Part model, mm, in its own coordinate system. Face numbers are marked on the shaded views. A direction names the side the tool comes from. Coordinates: 2 decimals unless noted, no trailing zeros. Write each loop counter-clockwise with the first axis right and the second up, starting at its lowest first coordinate (ties: lowest second). Pieces come first, ordered by that corner, then holes. Notation, with made-up numbers: (32, 55.5) -> (50, 55.5) arc R29 ccw to (50, 85.5) -> close; hole circle Ø1 at (-34, 85). An arc over 180 degrees is marked (long way). Write item = value, one per line.
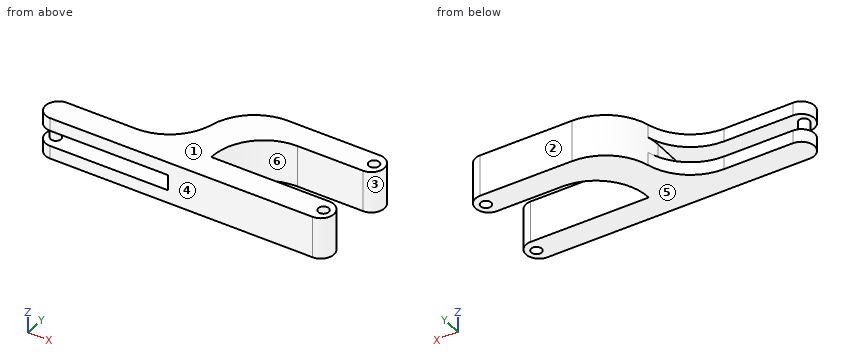
from build123d import *

# Parameters (mm, degrees)
SKETCH1_R           = 2
BOSS_EXTRUDE1_DEPTH = 8
SKETCH2_W           = 5
SKETCH2_H           = 10
BOSS_EXTRUDE2_DEPTH = 50
SKETCH3_R           = 2
BOSS_EXTRUDE3_DEPTH = 5
FILLET1_R           = 20
FILLET2_R           = 20
FILLET3_R           = 20
FILLET4_R           = 5


# Some blends are built 0.0001 mm under size
with BuildPart() as part:
    # Sketch1 → Boss-Extrude1 (new body)
    with BuildSketch(Plane.XY):
        Polygon((60, 20), (0, 20), (0, 0), (0, -20), (60, -20), (60, -10), (10, -10), (10, 0), (10, 10), (60, 10), align=None)
        with Locations((56, 15)):
            Circle(SKETCH1_R, mode=Mode.SUBTRACT)
        with Locations((56, -15)):
            Circle(SKETCH1_R, mode=Mode.SUBTRACT)
    boss_extrude1 = extrude(amount=BOSS_EXTRUDE1_DEPTH)

    # Sketch2 → Boss-Extrude2 (add)
    with BuildSketch(Plane.ZY):
        with Locations((5.5, -15)):
            Rectangle(SKETCH2_W, SKETCH2_H)
    boss_extrude2 = extrude(amount=BOSS_EXTRUDE2_DEPTH)

    # Sketch3 → Boss-Extrude3 (add)
    with BuildSketch(Plane(origin=(0, 0, 3), x_dir=(-1, 0, 0), z_dir=(0, 0, -1))):
        with Locations(Location((46, -15, 0), (0, 0, 270))):
            Circle(SKETCH3_R)
    boss_extrude3 = extrude(amount=BOSS_EXTRUDE3_DEPTH)

    # Mirror1: Boss-Extrude1, Boss-Extrude2, Boss-Extrude3 across plane
    add(boss_extrude1.mirror(Plane.XY))
    add(boss_extrude2.mirror(Plane.XY))
    add(boss_extrude3.mirror(Plane.XY))

    # Fillet1
    fillet1_edges = [part.edges().sort_by_distance(p)[0] for p in [
        (10, 10, 0),
    ]]
    fillet(fillet1_edges, radius=FILLET1_R - 0.0001)  # a hair under: the kernel refuses the full size

    # Fillet2
    fillet2_edges = [part.edges().sort_by_distance(p)[0] for p in [
        (0, 20, 0),
    ]]
    fillet(fillet2_edges, radius=FILLET2_R)

    # Fillet3
    # the kernel refuses this fillet: 20 mm, written as the material it adds along each edge
    with BuildSketch(Plane(origin=(0, -10, -43.824583655), x_dir=(0.042300987596812424, 0.9991049126334702, 0), z_dir=(0, 0, 1))) as fillet3_piece_1_section:
        with BuildLine():
            CenterArc((19.1898078, 19.559088377), FILLET3_R, 182.424391449, 75.522487814)
            Line((-0.792290453, 18.713068625), (-2.790500278, 18.62846665))
            Line((-2.790500278, 18.62846665), (-1.998209825, -0.084601975))
            Line((-1.998209825, -0.084601975), (0.084601975, -1.998209825))
            ThreePointArc((0.084601975, -1.998209825), (10.075651102, -1.575199949), (14.595801393, -1.955908838))
            Line((14.595801393, -1.955908838), (15.013438339, 0))
        make_face()
    fillet3_piece_1 = extrude(amount=98.64916731, mode=Mode.PRIVATE)
    fillet3_piece_1 = split(fillet3_piece_1, bisect_by=Plane(origin=(-6.457889851, -5.843011077, -8), z_dir=(0, 0, 1)), keep=Keep.TOP, mode=Mode.PRIVATE)
    fillet3_piece_1 = split(fillet3_piece_1, bisect_by=Plane(origin=(-6.457889851, -5.843011077, -3), z_dir=(0, 0, -1)), keep=Keep.TOP, mode=Mode.PRIVATE)
    add(fillet3_piece_1)
    with BuildSketch(Plane(origin=(0, -10, 3), x_dir=(0.042300987596807504, 0.9991049126334706, 0), z_dir=(0, 0, 1))) as fillet3_piece_2:
        with BuildLine():
            CenterArc((19.1898078, 19.559088377), FILLET3_R, 182.424391449, 75.522487814)
            Line((-0.792290453, 18.713068625), (-2.790500278, 18.62846665))
            Line((-2.790500278, 18.62846665), (-1.998209825, -0.084601975))
            Line((-1.998209825, -0.084601975), (0.084601975, -1.998209825))
            ThreePointArc((0.084601975, -1.998209825), (10.075651102, -1.575199949), (14.595801393, -1.955908838))
            Line((14.595801393, -1.955908838), (15.013438339, 0))
        make_face()
    extrude(amount=5)
    with BuildSketch(Plane(origin=(0, -10, 43.824583655), x_dir=(0.042300987596812424, 0.9991049126334702, 0), z_dir=(0, 0, -1))) as fillet3_piece_3_section:
        with BuildLine():
            CenterArc((19.1898078, -19.559088377), FILLET3_R, 102.053120737, 75.522487814)
            Line((-0.792290453, -18.713068625), (-2.790500278, -18.62846665))
            Line((-2.790500278, -18.62846665), (-1.998209825, 0.084601975))
            Line((-1.998209825, 0.084601975), (0.084601975, 1.998209825))
            ThreePointArc((0.084601975, 1.998209825), (10.075651102, 1.575199949), (14.595801393, 1.955908838))
            Line((14.595801393, 1.955908838), (15.013438339, 0))
        make_face()
    fillet3_piece_3 = extrude(amount=98.64916731, mode=Mode.PRIVATE)
    fillet3_piece_3 = split(fillet3_piece_3, bisect_by=Plane(origin=(-6.457889851, -5.843011077, 8), z_dir=(0, 0, -1)), keep=Keep.TOP, mode=Mode.PRIVATE)
    fillet3_piece_3 = split(fillet3_piece_3, bisect_by=Plane(origin=(-6.457889851, -5.843011077, 3), z_dir=(0, 0, 1)), keep=Keep.TOP, mode=Mode.PRIVATE)
    add(fillet3_piece_3)
    with BuildSketch(Plane(origin=(0, -10, -3), x_dir=(0.042300987596807504, 0.9991049126334706, 0), z_dir=(0, 0, -1))) as fillet3_piece_4:
        with BuildLine():
            CenterArc((19.1898078, -19.559088377), FILLET3_R, 102.053120737, 75.522487814)
            Line((-0.792290453, -18.713068625), (-2.790500278, -18.62846665))
            Line((-2.790500278, -18.62846665), (-1.998209825, 0.084601975))
            Line((-1.998209825, 0.084601975), (0.084601975, 1.998209825))
            ThreePointArc((0.084601975, 1.998209825), (10.075651102, 1.575199949), (14.595801393, 1.955908838))
            Line((14.595801393, 1.955908838), (15.013438339, 0))
        make_face()
    extrude(amount=5)
    # the kernel refuses this fillet: 20 mm, written as the material it takes off along each edge

    # Fillet4
    # the kernel refuses this fillet: 5 mm, written as the material it takes off along each edge
    with BuildSketch(Plane(origin=(60, 10, 20.5), x_dir=(0, 1, 0), z_dir=(0, 0, -1)), Plane(origin=(60, 20, 20.5), x_dir=(-1, 0, 0), z_dir=(0, 0, -1))) as fillet4_piece_1:
        with BuildLine():
            CenterArc((FILLET4_R, -FILLET4_R), FILLET4_R, 90, 90)
            Line((0, -FILLET4_R), (0, 0))
            Line((0, 0), (FILLET4_R, 0))
        make_face()
    extrude(amount=41, mode=Mode.SUBTRACT)
    with BuildSketch(Plane(origin=(60, -10, -20.5), x_dir=(-1, 0, 0), z_dir=(0, 0, 1)), Plane(origin=(60, -20, -20.5), x_dir=(0, 1, 0), z_dir=(0, 0, 1))) as fillet4_piece_2:
        with BuildLine():
            CenterArc((FILLET4_R, FILLET4_R), FILLET4_R, 180, 90)
            Line((0, FILLET4_R), (0, 0))
            Line((0, 0), (FILLET4_R, 0))
        make_face()
    extrude(amount=41, mode=Mode.SUBTRACT)
    with BuildSketch(Plane(origin=(-50, -10, -9.5), x_dir=(1, 0, 0), z_dir=(0, 0, 1)), Plane(origin=(-50, -10, 9.5), x_dir=(0, -1, 0), z_dir=(0, 0, -1))) as fillet4_piece_3:
        with BuildLine():
            CenterArc((FILLET4_R, -FILLET4_R), FILLET4_R, 90, 90)
            Line((0, -FILLET4_R), (0, 0))
            Line((0, 0), (FILLET4_R, 0))
        make_face()
    extrude(amount=30, mode=Mode.SUBTRACT)
    with BuildSketch(Plane(origin=(-50, -20, 20.5), x_dir=(0, 1, 0), z_dir=(0, 0, -1)), Plane(origin=(-50, -20, -20.5), x_dir=(1, 0, 0), z_dir=(0, 0, 1))) as fillet4_piece_4:
        with BuildLine():
            CenterArc((FILLET4_R, FILLET4_R), FILLET4_R, 180, 90)
            Line((0, FILLET4_R), (0, 0))
            Line((0, 0), (FILLET4_R, 0))
        make_face()
    extrude(amount=30, mode=Mode.SUBTRACT)


solid = part.part
Q1. Saw through at C-C on y = 15. Give the cut face in (x, z), and give its area (3 significant figures).
Model answer:
outline = (6.77, -8) -> (54, -8) -> (54, 8) -> (6.77, 8) -> close; (58, -8) -> (60, -8) -> (60, 8) -> (58, 8) -> close
area = 788 mm²
Q2. Pin check, flat tips, straight feed: pin 1 (1.5 mm diameter, centred on x = -29.5, z = 5, fed in from +Y); pin 2 (6.5 mm diameter, centred on y = -10, z = -1, fed in from -X); pin 3 (2 mm diameter, centred on y = -1.5, z = -6, fed in from -X). Stop position of each tip, or through.
Model answer:
pin_1 = -10
pin_2 = -49.37
pin_3 = -3.12
Q3. Mould opens along Y. For the marked faces 1, 2, 3 and 4 say: released by +Y, released by -Y, zero draft, split by the parting line, or undercut.
Model answer:
face_1 = zero draft
face_2 = released by +Y
face_3 = undercut
face_4 = released by -Y
Q4. Saw through at B-B on x = -21. Give the cut face in (y, z), and give its area (3 significant figures).
Model answer:
outline = (-20, -8) -> (-10, -8) -> (-10, -3) -> (-20, -3) -> close; (-20, 3) -> (-10, 3) -> (-10, 8) -> (-20, 8) -> close
area = 100 mm²
Q5. Which spindle directions (+Z, -Z, +X, -X, +Y, -Y) get a long thin tool onto all of the face, cutting with end or side? Do the marked faces 5 and 6. Say none if no direction does.
Model answer:
face_5 = -Z, +X, -X, +Y, -Y
face_6 = +Z, -Z, +X
Q6. Probe line 1 (Z direction, x = -20, y = -11); line 2 (X direction, y = -16, z = -2.25); line 3 (Y direction, x = 44, z = -4.75). List the from-to ranges inside material, lowest first. Write a range as from..to.
Model answer:
line_1 = -8..-3, 3..8
line_2 = -47.73..-44.27, 0..54.27, 57.73..59.9
line_3 = -20..-10, 10..20
Q7. Saw through at D-D on x = 56. Give the cut face in (y, z), and give its area (3 significant figures).
Model answer:
outline = (-19.9, -8) -> (-17, -8) -> (-17, 8) -> (-19.9, 8) -> close; (-13, -8) -> (-10.1, -8) -> (-10.1, 8) -> (-13, 8) -> close; (10.1, -8) -> (13, -8) -> (13, 8) -> (10.1, 8) -> close; (17, -8) -> (19.9, -8) -> (19.9, 8) -> (17, 8) -> close
area = 186 mm²
Q8. Saw through at A-A on z = 2. Count the separate pieces of the cut face and the enclosed holes in it, and give its area (3 significant figures).
Model answer:
separate_pieces = 2
enclosed_holes = 2
area = 1,370 mm²
